Check sheet for the modelled part. Datum: model origin and axes. Units: mm. A direction names the side the tool comes from. Give positions to 0.01 mm unless a question says otherwise; leave off trailing zeros. Order: outer loops, then holes, each group sorted by start corner. A loop starts at its lowest first (then second) coordinate and runs counter-clockwise, first axis right, second up. Notation, with made-up numbers: (12, 67.5) - (30, 67.5) arc R11 cw to (30, 81.5) - close; hole circle Ø2 at (5.5, -32). An arc over 180 degrees is marked (long way). Answer in a Markdown table with one row per item.
from build123d import *

# Parameters (mm, degrees)
F1_DEPTH = 2114


with BuildPart() as f1:
    # F0 (on Right) → F1 (new body)
    with BuildSketch(Plane.YZ):
        with BuildLine():
            ThreePointArc((0, 4), (1.171573, 1.171573), (4, 0))
            Line((4, 0), (40, 0))
            Line((40, 0), (40, 4))
            Line((40, 4), (8, 4))
            ThreePointArc((8, 4), (5.171573, 5.171573), (4, 8))
            Line((4, 8), (4, 146))
            ThreePointArc((4, 146), (5.171573, 148.828427), (8, 150))
            Line((8, 150), (52, 150))
            ThreePointArc((52, 150), (54.828427, 148.828427), (56, 146))
            Line((56, 146), (56, 122))
            ThreePointArc((56, 122), (57.171573, 119.171573), (60, 118))
            Line((60, 118), (100, 118))
            Line((100, 118), (100, 122))
            Line((100, 122), (64, 122))
            ThreePointArc((64, 122), (61.171573, 123.171573), (60, 126))
            Line((60, 126), (60, 150))
            ThreePointArc((60, 150), (58.828427, 152.828427), (56, 154))
            Line((56, 154), (4, 154))
            ThreePointArc((4, 154), (1.171573, 152.828427), (0, 150))
            Line((0, 150), (0, 4))
        make_face()
    extrude(amount=F1_DEPTH)


solid = f1.part
(1) Cross-section at C-C, the plane y = 83.5. Record the cut outline in (x, z), then the cut area to 3 significant figures.
Geometry says:
| item | result |
|---|---|
| outline | (0, 118) - (2114, 118) - (2114, 122) - (0, 122) - close |
| area | 8,460 mm² |
(2) Access from +Z, -Z, +X, -X, +Y, -Y to the whole of each face (thin tool, end or side, straight path). Record for faces 4 (the flat face through (2114, 2, 89)), 5 (the flat face through (1042, 82, 122)), 6 (the flat face through (1042, 24, 4)), 7 (the flat face through (1042, 4, 76)).
Geometry says:
| item | result |
|---|---|
| face 4 | +Z, -Z, +X, +Y, -Y |
| face 5 | +Z, +X, -X, +Y |
| face 6 | +X, -X, +Y |
| face 7 | +X, -X |
(3) Cross-section at A-A, the plane x = 1532. Record the cut outline in (y, z).
Geometry says:
| item | result |
|---|---|
| outline | (0, 4) arc R4 ccw to (4, 0) - (40, 0) - (40, 4) - (8, 4) arc R4 cw to (4, 8) - (4, 146) arc R4 cw to (8, 150) - (52, 150) arc R4 cw to (56, 146) - (56, 122) arc R4 ccw to (60, 118) - (100, 118) - (100, 122) - (64, 122) arc R4 cw to (60, 126) - (60, 150) arc R4 ccw to (56, 154) - (4, 154) arc R4 ccw to (0, 150) - close |
(4) Gauge pin test, flat ends, axial feed: P1, Ø5, axis at x = 1829, y = 74, coming from the +Z side; P2, Ø6, axis at x = 1006, y = 80.5, coming from the -Z side; P3, Ø2, axis at x = 1168, z = 1.5, coming from the +Y side. Record the tip position at first contact, or that the pin passes through.
Geometry says:
| item | result |
|---|---|
| P1 | z = 122 |
| P2 | z = 118 |
| P3 | y = 40 |
(5) Mould release check, pull along Z, two halves, no side actions. Record for faces 1 (the flat face through (1042, 30, 150)), 2 (the flat face through (1042, 0, 78)), 3 (the flat face through (1042, 80, 118)): pulls with the +Z half, pulls with the -Z half, needs draft (parallel to the pull), parting line crosses it, or undercut.
Geometry says:
| item | result |
|---|---|
| face 1 | undercut |
| face 2 | needs draft |
| face 3 | pulls with the -Z half |
(6) Thickness scan on L1, parallel to Z at x = 861.5, y = 13; L2, parallel to Y at x = 1204, z = 69; L3, parallel to Y at x = 453.5, z = 130.5. Record the ranges inside material, lowest first.
Geometry says:
| item | result |
|---|---|
| L1 | 0 to 4, 150 to 154 |
| L2 | 0 to 4 |
| L3 | 0 to 4, 56 to 60 |
(7) Cross-section at B-B, the plane z = 60. Record the cut outline in (x, y).
Geometry says:
| item | result |
|---|---|
| outline | (0, 0) - (2114, 0) - (2114, 4) - (0, 4) - close |
